Read the model definition and answer for the solid it produces. Units are mm, in the model's axes. Give positions to 0.01 mm unless a question says otherwise; leave off trailing zeros. Write each loop counter-clockwise with the first axis right and the second up, starting at its lowest first coordinate (ties: lowest second). Pieces come first, ordered by that corner, then holes. Notation, with made-up numbers: (79, 35) -> (132, 35) arc R8 cw to (132, 46) -> close; hole circle Ø5 at (60.25, 15). An arc over 180 degrees is marked (long way). Answer as CSV lines item,"result". Start each with the question number.
1. The part is cut by section B-B, the plane x = 4.5. Determine the outline of the cut face in (y, z) (3 decimals).
2. The part is cut by section A-A, the plane y = 38.1. Determine the outline of the cut face in (x, z) (3 decimals), and give its area (3 significant figures).
3. Given pin 1 (4 mm diameter, centred on y = -16.5, z = -8, fed in from -X); pin 2 (4 mm diameter, centred on y = 0, z = 0, fed in from +X), each flat-ended and moving along its own axis, determine where each tip first touches the part or whether it passes through.
4. Find the intervals of material crossed by line 1 (Z direction, x = 2.5, y = 0) (3 decimals); line 2 (Y direction, x = 5.25, z = -1); line 3 (Z direction, x = 4.25, y = 39), in increasing order.
5. For a pull along Z with two mould halves and no side action, classify faces 1 (the flat face through (3, 101.6, 0)), 2 (the flat face through (3, -1, -25.4)), 3 (the cylindrical face through (3.13, -41.27, 0.14)) as pulls with the +Z half, pulls with the -Z half, needs draft (parallel to the pull), parting line crosses it, or undercut.
6. The part is cut by section C-C, the plane z = 0. Determine the outline of the cut face in (x, y) (3 decimals).
from build123d import *

# Parameters (mm, degrees)
F0_W     = 203.2
F0_H     = 50.8
F0_R     = 3.175
F1_DEPTH = 6.35


with BuildPart() as f1:
    # F0 (on Right) → F1 (new body)
    with BuildSketch(Plane.YZ):
        Rectangle(F0_W, F0_H)
        with Locations((-76.2, 0)):
            Circle(F0_R, mode=Mode.SUBTRACT)
        with Locations((-38.1, 0)):
            Circle(F0_R, mode=Mode.SUBTRACT)
        Circle(F0_R, mode=Mode.SUBTRACT)
        with Locations((38.1, 0)):
            Circle(F0_R, mode=Mode.SUBTRACT)
        with Locations((76.2, 0)):
            Circle(F0_R, mode=Mode.SUBTRACT)
    extrude(amount=F1_DEPTH)


solid = f1.part
Results found:
1,outline,"(-101.6, -25.4) -> (101.6, -25.4) -> (101.6, 25.4) -> (-101.6, 25.4) -> close; hole circle Ø6.35 at (-76.2, 0); hole circle Ø6.35 at (-38.1, 0); hole circle Ø6.35 at (0, 0); hole circle Ø6.35 at (38.1, 0); hole circle Ø6.35 at (76.2, 0)"
2,outline,"(0, -25.4) -> (6.35, -25.4) -> (6.35, -3.175) -> (0, -3.175) -> close; (0, 3.175) -> (6.35, 3.175) -> (6.35, 25.4) -> (0, 25.4) -> close"
2,area,"282 mm²"
3,pin 1,"stops at x = 0"
3,pin 2,"passes through"
4,line 1,"z = -25.4 to -3.175, 3.175 to 25.4"
4,line 2,"y = -101.6 to -79.21, -73.19 to -41.11, -35.09 to -3.01, 3.01 to 35.09, 41.11 to 73.19, 79.21 to 101.6"
4,line 3,"z = -25.4 to -3.04, 3.04 to 25.4"
5,face 1,"needs draft"
5,face 2,"pulls with the -Z half"
5,face 3,"undercut"
6,outline,"(0, -101.6) -> (6.35, -101.6) -> (6.35, -79.375) -> (0, -79.375) -> close; (0, -73.025) -> (6.35, -73.025) -> (6.35, -41.275) -> (0, -41.275) -> close; (0, -34.925) -> (6.35, -34.925) -> (6.35, -3.175) -> (0, -3.175) -> close; (0, 3.175) -> (6.35, 3.175) -> (6.35, 34.925) -> (0, 34.925) -> close; (0, 41.275) -> (6.35, 41.275) -> (6.35, 73.025) -> (0, 73.025) -> close; (0, 79.375) -> (6.35, 79.375) -> (6.35, 101.6) -> (0, 101.6) -> close"
